For this review, take the finished solid that the model builds, in its own axes (mm). Face numbers are marked on the shaded views. Give positions to 0.01 mm unless a question says otherwise; leave off trailing zeros. Write each loop counter-clockwise with the first axis right and the second up, starting at its lowest first coordinate (ties: lowest second). Pieces come first, ordered by that corner, then holes.
1) We need section B-B on y = 19.5. Give the boundary of the cut face in (x, z), and give its area (3 significant figures).
2) Wall thickness on line 1 along Y through (x, z) = (32, 6.5); line 2 along Y through (x, z) = (40.5, 1); line 3 along X through (y, z) = (-33.5, 7.25): over which ranges is each line inside the solid? List them lowest first.
3) For P1, Ø5, axis at x = 31, z = 4.5, coming from the +Y side; P2, Ø5, axis at y = -32, z = 5, coming from the -X side; P3, Ø5, axis at x = 33.5, z = 6.5, coming from the +Y side, all flat-tipped, find the tip position at first contact; note any pin that passes through.
4) We need section A-A on x = -37.5. Give the boundary of the cut face in (y, z), and give its area (3 significant figures).
5) Draft analysis for pull direction X (two halves, no side actions). For the marked faces 1, 2 and 3, state which applies: pulls with the +X half, pulls with the -X half, needs draft (parallel to the pull), parting line crosses it, or undercut.
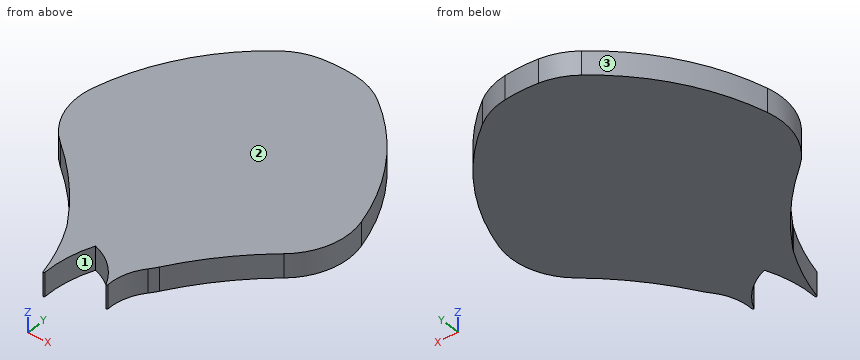
from build123d import *

# Parameters (mm, degrees)
F1_DEPTH    = 9
F2_DEPTH    = 9
F3_T1_DEPTH = 9
F3_T3_DEPTH = 97.7984007527
F3_T5_DEPTH = 18.7464853336
F3_T7_DEPTH = 44.8077335821
F4_F1_R     = 0.3
F4_F2_R     = 0.3


# Not quite as in the source:
# - a fillet or chamfer that OpenCascade refuses, or shapes differently, is made with other operations: its cross-section is extruded or revolved along the edge and cut away or added


with BuildPart() as f1:
    # F0 (on Top) → F1 (new body)
    with BuildSketch(Plane.XY):
        with BuildLine():
            ThreePointArc((52.3559108968, -15.2742949835), (41.1175441228, 23.5793695766), (13.2592789192, 52.9021456617))
            ThreePointArc((13.2592789192, 52.9021456617), (0, 54.5384771796), (-13.2592789192, 52.9021456617))
            ThreePointArc((-13.2592789192, 52.9021456617), (-41.1175441228, 23.5793695766), (-52.3559108968, -15.2742949835))
            ThreePointArc((-52.3559108968, -15.2742949835), (-32.1035122758, -31.703635387), (-15.9292943442, -52.1603592277))
            ThreePointArc((-15.9292943442, -52.1603592277), (-9.8139264878, -53.648227743), (-3.5678639787, -54.4216486309))
            ThreePointArc((-3.5678639787, -54.4216486309), (6.2832792085, -54.1753255224), (15.9292943442, -52.1603592277))
            ThreePointArc((15.9292943442, -52.1603592277), (32.1035122758, -31.703635387), (52.3559108968, -15.2742949835))
        make_face()
    extrude(amount=F1_DEPTH)

    # F0 (on Top) → F2 (join)
    with BuildSketch(Plane.XY):
        with BuildLine():
            ThreePointArc((-7.0224064402, -78.6131843925), (-7.0174520358, -66.2714702986), (-3.5678639787, -54.4216486309))
            ThreePointArc((-3.5678639787, -54.4216486309), (-9.8139264878, -53.648227743), (-15.9292943442, -52.1603592277))
            ThreePointArc((-15.9292943442, -52.1603592277), (-10.336712225, -65.0032144434), (-7.0224064402, -78.6131843925))
        make_face()
        with BuildLine():
            ThreePointArc((10.5660464615, -68.2554319501), (11.3560818324, -59.5775748336), (15.9292943442, -52.1603592277))
            ThreePointArc((15.9292943442, -52.1603592277), (6.2832792085, -54.1753255224), (-3.5678639787, -54.4216486309))
            ThreePointArc((-3.5678639787, -54.4216486309), (5.1525036315, -59.6492567371), (10.5660464615, -68.2554319501))
        make_face()
    extrude(amount=F2_DEPTH)

    # F3: fillet of radius 25 on 6 edges, made by hand

    # F3_s2 → F3_t1 (join)
    with BuildSketch(Plane.XY):
        with BuildLine():
            ThreePointArc((-16.4732265546, -51.2989033705), (-15.9263980679, -52.1979676734), (-15.4178890795, -53.1192475566))
            ThreePointArc((-15.4178890795, -53.1192475566), (-15.6719958304, -52.6389522584), (-15.9292943442, -52.1603592277))
            ThreePointArc((-15.9292943442, -52.1603592277), (-16.2003358533, -51.7290474995), (-16.4732265546, -51.2989033705))
        make_face()
    extrude(amount=F3_T1_DEPTH)

    # F3_s4 → F3_t3 (cut)
    with BuildSketch(Plane.XY.offset(-44.3992003763)):
        with BuildLine():
            ThreePointArc((41.3774463504, -23.2564339871), (49.2973579438, -11.704046911), (49.7610601076, 2.2947968664))
            ThreePointArc((49.7610601076, 2.2947968664), (51.5165033775, -6.4221025316), (52.3559108968, -15.2742949835))
            ThreePointArc((52.3559108968, -15.2742949835), (46.752445175, -19.108250225), (41.3774463504, -23.2564339871))
        make_face()
        with BuildLine():
            ThreePointArc((-49.7610601076, 2.2947968664), (-49.2973579438, -11.704046911), (-41.3774463504, -23.2564339871))
            ThreePointArc((-41.3774463504, -23.2564339871), (-46.752445175, -19.108250225), (-52.3559108968, -15.2742949835))
            ThreePointArc((-52.3559108968, -15.2742949835), (-51.5165033775, -6.4221025316), (-49.7610601076, 2.2947968664))
        make_face()
    extrude(amount=F3_T3_DEPTH, mode=Mode.SUBTRACT)

    # F3_s6 → F3_t5 (cut)
    with BuildSketch(Plane.XY.offset(-4.8732426668)):
        with BuildLine():
            ThreePointArc((16.9764615861, -50.5162181687), (16.0190019724, -51.8895795654), (14.9717711174, -53.195779387))
            ThreePointArc((14.9717711174, -53.195779387), (15.4409431776, -52.6692011973), (15.9292943442, -52.1603592277))
            ThreePointArc((15.9292943442, -52.1603592277), (16.4495016002, -51.3361382631), (16.9764615861, -50.5162181687))
        make_face()
    extrude(amount=F3_T5_DEPTH, mode=Mode.SUBTRACT)

    # F3_s8 → F3_t7 (cut)
    with BuildSketch(Plane.XY.offset(-17.903866791)):
        with BuildLine():
            ThreePointArc((18.4012083068, 49.3190772564), (12.6321038646, 52.5652026084), (6.2132770502, 54.1833985771))
            ThreePointArc((6.2132770502, 54.1833985771), (9.7573311543, 53.6585499414), (13.2592789192, 52.9021456617))
            ThreePointArc((13.2592789192, 52.9021456617), (15.8631283238, 51.1578030954), (18.4012083068, 49.3190772564))
        make_face()
        with BuildLine():
            ThreePointArc((-6.2132770502, 54.1833985771), (-12.6321038646, 52.5652026084), (-18.4012083068, 49.3190772564))
            ThreePointArc((-18.4012083068, 49.3190772564), (-15.8631283238, 51.1578030954), (-13.2592789192, 52.9021456617))
            ThreePointArc((-13.2592789192, 52.9021456617), (-9.7573311543, 53.6585499414), (-6.2132770502, 54.1833985771))
        make_face()
    extrude(amount=F3_T7_DEPTH, mode=Mode.SUBTRACT)

    # F4: fillet of radius 0.3 on 2 edges, made by hand

    # F4_f1
    f4_f1_edges = [f1.edges().sort_by_distance(p)[0] for p in [
        (-7.0224064402, -78.6131843925, 4.5),
    ]]
    fillet(f4_f1_edges, radius=F4_F1_R)

    # F4_f2
    f4_f2_edges = [f1.edges().sort_by_distance(p)[0] for p in [
        (10.5660464615, -68.2554319501, 4.5),
    ]]
    fillet(f4_f2_edges, radius=F4_F2_R)


solid = f1.part
Results list:
1. outline: (-43.31, 0) - (43.31, 0) - (43.31, 9) - (-43.31, 9) - close
1. area: 780 mm2
2. line 1: y = -31.81 to 36.53
2. line 2: y = -23.98 to 24.64
2. line 3: x = -30.37 to 30.37
3. P1: stops at y = 40.38
3. P2: stops at x = -34.34
3. P3: stops at y = 37.68
4. outline: (-26.57, 0) - (29.34, 0) - (29.34, 9) - (-26.57, 9) - close
4. area: 503 mm2
5. face 1: undercut
5. face 2: needs draft
5. face 3: pulls with the -X half
